Geometry: see drawing. Coordinates: mm, zero at the bounding-box minimum. A direction names the side the tool comes from. Give positions to 0.01 mm unless a question says otherwise; leave off trailing zeros. Write each loop counter-clockwise with the first axis right and the second up, starting at its lowest first coordinate (ties: lowest second). Pieces come first, ordered by that corner, then holes. Notation, with made-up numbers: M 33,50 L 73,50 A18 cw 73,83 Z; hole C 70.5,50.5 d6. An arc over 180 degrees is marked long. Use CSV: the item, a comma, the result in double quotes. Start each with the question number.
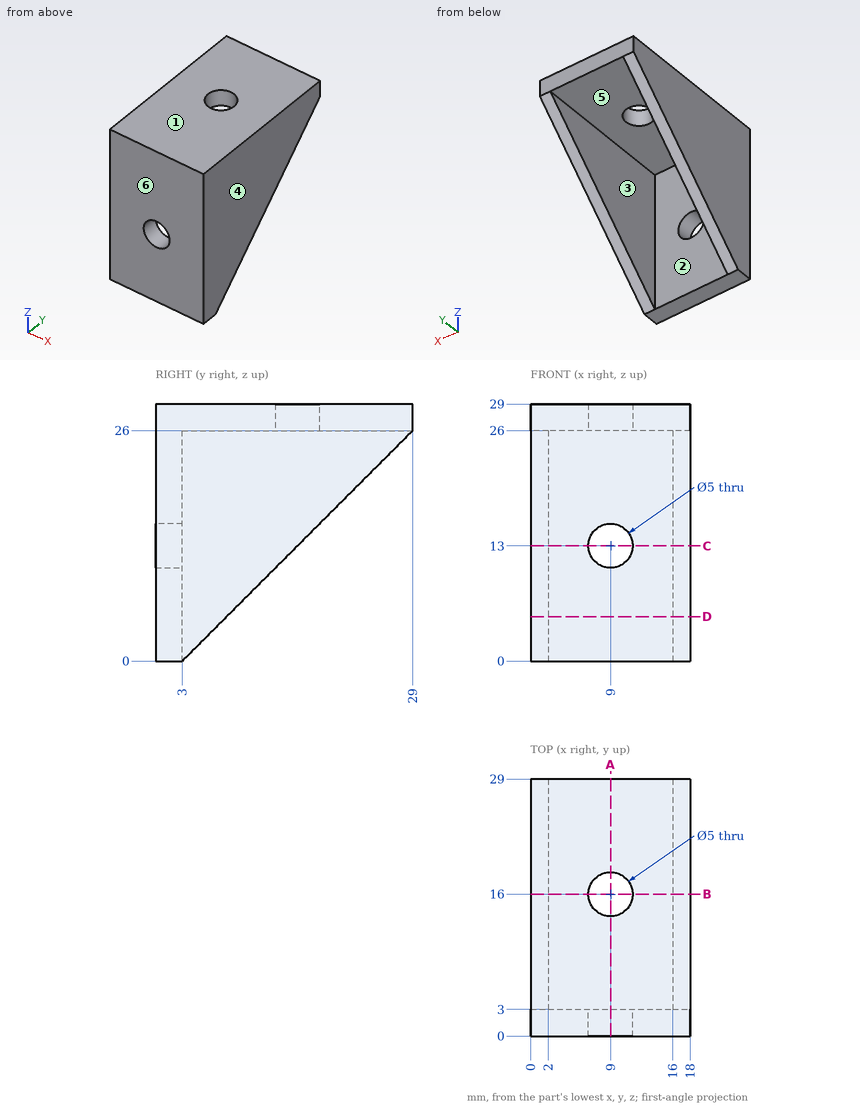
1. Section B-B on y = 16. Return loops of the section in (x, z).
2. Section D-D on z = 5. Return loops of the section in (x, y).
3. Line query: probe 1 along X at (y, z) = (13.25, 25); probe 2 along X at (y, z) = (16, 27.2); probe 3 along Z at (x, y) = (4, 6.25). Output: solid intervals per line, ascending.
4. Section C-C on z = 13. Return loops of the section in (x, y).
5. Access query for the marked faces 5 and 6. Directions: +Z, -Z, +X, -X, +Y, -Y. A direction counts if a zero-diameter tool reaches every point of the face in a straight line with its end or side. Return the directions, or none.
6. First-contact query: pin 1 (8 mm diameter, centred on x = 9, z = 13, fed in from +Y); pin 2 (4 mm diameter, centred on x = 11, y = 16, fed in from -Z). Flat tips, straight axial feed; report the tip coordinate or a pass-through.
7. Pull-direction query (X, two-part tool) for the marked faces 1, 2, 3 and 4; classes: released by +X, released by -X, zero draft, split by the parting line, or undercut.
8. Section A-A on x = 9. Return loops of the section in (y, z), then the cut area to 3 significant figures.
Resolved:
1,outline,"M 0,13 L 2,13 L 2,26 L 6.5,26 L 6.5,29 L 0,29 Z; M 11.5,26 L 16,26 L 16,13 L 18,13 L 18,29 L 11.5,29 Z"
2,outline,"M 0,0 L 18,0 L 18,8 L 16,8 L 16,3 L 2,3 L 2,8 L 0,8 Z"
3,probe 1,"x = 0 to 2, 16 to 18"
3,probe 2,"x = 0 to 6.5, 11.5 to 18"
3,probe 3,"z = 26 to 29"
4,outline,"M 0,0 L 6.5,0 L 6.5,3 L 2,3 L 2,16 L 0,16 Z; M 11.5,0 L 18,0 L 18,16 L 16,16 L 16,3 L 11.5,3 Z"
5,face 5,"-Z, +Y"
5,face 6,"+Z, -Z, +X, -X, -Y"
6,pin 1,"stops at y = 3"
6,pin 2,"stops at z = 26"
7,face 1,"zero draft"
7,face 2,"undercut"
7,face 3,"undercut"
7,face 4,"released by +X"
8,outline,"M 0,0 L 3,0 L 3,10.5 L 0,10.5 Z; M 0,15.5 L 3,15.5 L 3,26 L 13.5,26 L 13.5,29 L 0,29 Z; M 18.5,26 L 29,26 L 29,29 L 18.5,29 Z"
8,area,"135 mm2"
